from build123d import *

# Parameters (mm, degrees)
F1_DEPTH     = 25
F2_T         = 2
F3_T1_DEPTH  = 31
F3_T3_DEPTH  = 46
F3_T9_DEPTH  = 51
F3_T13_DEPTH = 36
F3_T20_DEPTH = 36
F3_T24_DEPTH = 51
F3_T31_DEPTH = 36
F3_T35_DEPTH = 51
F3_T42_DEPTH = 36
F3_T46_DEPTH = 51
F4_R         = 3
F5_R         = 1
F6_DEPTH     = 4
F8_W         = 10
F8_H         = 4
F9_DEPTH     = 4


# Not quite as in the source:
# - a fillet or chamfer that OpenCascade refuses, or shapes differently, is made with other operations: its cross-section is extruded or revolved along the edge and cut away or added
# - a shell that OpenCascade refuses in one call is made with other operations: the cavity is built on its own and cut out


with BuildPart() as f1:
    # F0 (on Top) → F1 (new body)
    with BuildSketch(Plane.XY):
        with BuildLine():
            ThreePointArc((25, 15.5), (24.4142135624, 16.9142135624), (23, 17.5))
            Line((23, 17.5), (-23, 17.5))
            ThreePointArc((-23, 17.5), (-24.4142135624, 16.9142135624), (-25, 15.5))
            Line((-25, 15.5), (-25, -15.5))
            ThreePointArc((-25, -15.5), (-24.4142135624, -16.9142135624), (-23, -17.5))
            Line((-23, -17.5), (23, -17.5))
            ThreePointArc((23, -17.5), (24.4142135624, -16.9142135624), (25, -15.5))
            Line((25, -15.5), (25, 15.5))
        make_face()
    extrude(amount=F1_DEPTH)

    # F2: shell of thickness 2, made by hand


with BuildPart() as f2_core1:
    # F2_t2: copy of F1
    add(f1.part)

    # the walls: a layer under each face that stays
    f2_faces = [f2_core1.faces().sort_by_distance(p)[0] for p in [
        (0, 17.5, 12.5),
        (-25, 0, 12.5),
        (0, -17.5, 12.5),
        (25, 0, 12.5),
        (0, 0, 0),
    ]]
    thicken(f2_faces, amount=-F2_T, mode=Mode.SUBTRACT)


with BuildPart() as f1_1:
    add(f1.part)

    # what is left inside the walls is the cavity
    f2_cavity = [f2_core1.part.solids().sort_by_distance(p)[0] for p in [
        (0, -5.166667, 2.02),
    ]]
    add(f2_cavity, mode=Mode.SUBTRACT)

    # F3: fillet of radius 2 on 4 edges, made by hand

    # F3_s2 → F3_t1 (cut)
    with BuildSketch(Plane.XZ.offset(-15.5)):
        with BuildLine():
            ThreePointArc((-25, 25), (-23.5857864376, 24.4142135624), (-23, 23))
            Line((-23, 23), (-22.96, 23))
            Line((-22.96, 23), (-22.96, 25.04))
            Line((-22.96, 25.04), (-25, 25.04))
            Line((-25, 25.04), (-25, 25))
        make_face()
        with BuildLine():
            ThreePointArc((25, 25), (23.5857864376, 24.4142135624), (23, 23))
            Line((23, 23), (22.96, 23))
            Line((22.96, 23), (22.96, 25.04))
            Line((22.96, 25.04), (25, 25.04))
            Line((25, 25.04), (25, 25))
        make_face()
    extrude(amount=F3_T1_DEPTH, mode=Mode.SUBTRACT)

    # F3_s4 → F3_t3 (cut)
    with BuildSketch(Plane.YZ.offset(-23)):
        with BuildLine():
            ThreePointArc((17.5, 25), (16.0857864376, 24.4142135624), (15.5, 23))
            Line((15.5, 23), (15.46, 23))
            Line((15.46, 23), (15.46, 25.04))
            Line((15.46, 25.04), (17.5, 25.04))
            Line((17.5, 25.04), (17.5, 25))
        make_face()
        with BuildLine():
            ThreePointArc((-17.5, 25), (-16.0857864376, 24.4142135624), (-15.5, 23))
            Line((-15.5, 23), (-15.46, 23))
            Line((-15.46, 23), (-15.46, 25.04))
            Line((-15.46, 25.04), (-17.5, 25.04))
            Line((-17.5, 25.04), (-17.5, 25))
        make_face()
    extrude(amount=F3_T3_DEPTH, mode=Mode.SUBTRACT)


with BuildPart() as f3_tool7:
    # F3_s8 → F3_t9 (new body)
    with BuildSketch(Plane.YZ.offset(23)):
        with BuildLine():
            ThreePointArc((17.5, 25), (16.0857864376, 24.4142135624), (15.5, 23))
            Line((15.5, 23), (15.46, 23))
            Line((15.46, 23), (15.46, 25.04))
            Line((15.46, 25.04), (17.5, 25.04))
            Line((17.5, 25.04), (17.5, 25))
        make_face()
    extrude(amount=-F3_T9_DEPTH)

    split(bisect_by=Plane.YZ.offset(-23), keep=Keep.BOTTOM)


with BuildPart() as f3_tool11:
    # F3_s12 → F3_t13 (new body)
    with BuildSketch(Plane.XZ.offset(-20.5)):
        with BuildLine():
            ThreePointArc((-25, 25), (-23.5857864376, 24.4142135624), (-23, 23))
            Line((-23, 23), (-22.96, 23))
            Line((-22.96, 23), (-22.96, 25.04))
            Line((-22.96, 25.04), (-25, 25.04))
            Line((-25, 25.04), (-25, 25))
        make_face()
    extrude(amount=F3_T13_DEPTH)

    split(bisect_by=Plane.XZ.offset(-15.5), keep=Keep.BOTTOM)


with BuildPart() as f3_tool7_1:
    add(f3_tool7.part)

    # F3_t15: intersect F3_tool11
    add(f3_tool11.part, mode=Mode.INTERSECT)


with BuildPart() as f1_2:
    add(f1_1.part)

    # F3_t5: cut F3_tool7
    add(f3_tool7_1.part, mode=Mode.SUBTRACT)


with BuildPart() as f3_tool18:
    # F3_s19 → F3_t20 (new body)
    with BuildSketch(Plane.XZ.offset(-15.5)):
        with BuildLine():
            ThreePointArc((-25, 25), (-23.5857864376, 24.4142135624), (-23, 23))
            Line((-23, 23), (-22.96, 23))
            Line((-22.96, 23), (-22.96, 25.04))
            Line((-22.96, 25.04), (-25, 25.04))
            Line((-25, 25.04), (-25, 25))
        make_face()
    extrude(amount=F3_T20_DEPTH)

    split(bisect_by=Plane.XZ.offset(15.5), keep=Keep.TOP)


with BuildPart() as f3_tool22:
    # F3_s23 → F3_t24 (new body)
    with BuildSketch(Plane.YZ.offset(-28)):
        with BuildLine():
            ThreePointArc((-17.5, 25), (-16.0857864376, 24.4142135624), (-15.5, 23))
            Line((-15.5, 23), (-15.46, 23))
            Line((-15.46, 23), (-15.46, 25.04))
            Line((-15.46, 25.04), (-17.5, 25.04))
            Line((-17.5, 25.04), (-17.5, 25))
        make_face()
    extrude(amount=F3_T24_DEPTH)

    split(bisect_by=Plane.YZ.offset(-23), keep=Keep.BOTTOM)


with BuildPart() as f3_tool18_1:
    add(f3_tool18.part)

    # F3_t26: intersect F3_tool22
    add(f3_tool22.part, mode=Mode.INTERSECT)


with BuildPart() as f1_3:
    add(f1_2.part)

    # F3_t16: cut F3_tool18
    add(f3_tool18_1.part, mode=Mode.SUBTRACT)


with BuildPart() as f3_tool29:
    # F3_s30 → F3_t31 (new body)
    with BuildSketch(Plane.XZ.offset(15.5)):
        with BuildLine():
            ThreePointArc((25, 25), (23.5857864376, 24.4142135624), (23, 23))
            Line((23, 23), (22.96, 23))
            Line((22.96, 23), (22.96, 25.04))
            Line((22.96, 25.04), (25, 25.04))
            Line((25, 25.04), (25, 25))
        make_face()
    extrude(amount=-F3_T31_DEPTH)

    split(bisect_by=Plane.XZ.offset(-15.5), keep=Keep.BOTTOM)


with BuildPart() as f3_tool33:
    # F3_s34 → F3_t35 (new body)
    with BuildSketch(Plane.YZ.offset(28)):
        with BuildLine():
            ThreePointArc((17.5, 25), (16.0857864376, 24.4142135624), (15.5, 23))
            Line((15.5, 23), (15.46, 23))
            Line((15.46, 23), (15.46, 25.04))
            Line((15.46, 25.04), (17.5, 25.04))
            Line((17.5, 25.04), (17.5, 25))
        make_face()
    extrude(amount=-F3_T35_DEPTH)

    split(bisect_by=Plane.YZ.offset(23), keep=Keep.TOP)


with BuildPart() as f3_tool29_1:
    add(f3_tool29.part)

    # F3_t37: intersect F3_tool33
    add(f3_tool33.part, mode=Mode.INTERSECT)


with BuildPart() as f1_4:
    add(f1_3.part)

    # F3_t27: cut F3_tool29
    add(f3_tool29_1.part, mode=Mode.SUBTRACT)


with BuildPart() as f3_tool40:
    # F3_s41 → F3_t42 (new body)
    with BuildSketch(Plane.XZ.offset(20.5)):
        with BuildLine():
            ThreePointArc((25, 25), (23.5857864376, 24.4142135624), (23, 23))
            Line((23, 23), (22.96, 23))
            Line((22.96, 23), (22.96, 25.04))
            Line((22.96, 25.04), (25, 25.04))
            Line((25, 25.04), (25, 25))
        make_face()
    extrude(amount=-F3_T42_DEPTH)

    split(bisect_by=Plane.XZ.offset(15.5), keep=Keep.TOP)


with BuildPart() as f3_tool44:
    # F3_s45 → F3_t46 (new body)
    with BuildSketch(Plane.YZ.offset(-23)):
        with BuildLine():
            ThreePointArc((-17.5, 25), (-16.0857864376, 24.4142135624), (-15.5, 23))
            Line((-15.5, 23), (-15.46, 23))
            Line((-15.46, 23), (-15.46, 25.04))
            Line((-15.46, 25.04), (-17.5, 25.04))
            Line((-17.5, 25.04), (-17.5, 25))
        make_face()
    extrude(amount=F3_T46_DEPTH)

    split(bisect_by=Plane.YZ.offset(23), keep=Keep.TOP)


with BuildPart() as f3_tool40_1:
    add(f3_tool40.part)

    # F3_t48: intersect F3_tool44
    add(f3_tool44.part, mode=Mode.INTERSECT)


with BuildPart() as f1_5:
    add(f1_4.part)

    # F3_t38: cut F3_tool40
    add(f3_tool40_1.part, mode=Mode.SUBTRACT)

    # F4
    f4_edges = [f1_5.edges().sort_by_distance(p)[0] for p in [
        (0, 15.5, 2),
        (23, 0, 2),
        (0, -15.5, 2),
        (-23, 0, 2),
    ]]
    fillet(f4_edges, radius=F4_R)

    # F5 (on Top) → F6 (join)
    with BuildSketch(Plane.XY):
        with Locations((-9, 4.5)):
            Circle(F5_R)
        with Locations((-9, -5.5)):
            Circle(F5_R)
        with Locations((9, 4.5)):
            Circle(F5_R)
        with Locations((9, -5.5)):
            Circle(F5_R)
    extrude(amount=F6_DEPTH)

    # F8 (on offset) → F9 (cut, symmetric)
    with BuildSketch(Plane.YZ.offset(23.5)):
        with Locations((0, 6)):
            Rectangle(F8_W, F8_H)
    extrude(amount=F9_DEPTH, both=True, mode=Mode.SUBTRACT)


solid = f1_5.part
Part model, mm, in its own coordinate system. A direction names the side the tool comes from. Round coordinates to 2 decimals unless told otherwise and drop trailing zeros. Loops run counter-clockwise (first coordinate to the right, second up) from the corner with the lowest first, then second, coordinate; pieces in that order, holes last. Notation, with made-up numbers: (29.5, 56) - (71.5, 56) arc R20 ccw to (71.5, 60) - close; hole circle Ø1 at (2, 52.5). An arc over 180 degrees is marked (long way). Answer as a JSON object with one key per item and string values.
Item 1: Pull direction X, two halves, no side cores. Call faces 4 (the face through (0.34, 16.1, 24.43)), 5 (the face through (-24.4, 16.93, 12.33)), 6 (the face through (25, 0, 12)): pulls with the +X half, pulls with the -X half, needs draft (parallel to the pull), parting line crosses it, or undercut.
Output:
{"face 4": "undercut", "face 5": "pulls with the -X half", "face 6": "pulls with the +X half"}
Item 2: Band-saw the part on D-D on y = 11. List the corners of the cut face in (x, z).
Output:
{"outline": "(-25, 0) - (25, 0) - (25, 25) arc R2 ccw to (23, 23) - (23, 5) arc R3 cw to (20, 2) - (-20, 2) arc R3 cw to (-23, 5) - (-23, 23) arc R2 ccw to (-25, 25) - close"}
Item 3: Band-saw the part on B-B on z = 13.5. List the corners of the cut face in (x, y).
Output:
{"outline": "(-25, -15.5) arc R2 ccw to (-23, -17.5) - (23, -17.5) arc R2 ccw to (25, -15.5) - (25, 15.5) arc R2 ccw to (23, 17.5) - (-23, 17.5) arc R2 ccw to (-25, 15.5) - close; hole (-23, -15.5) - (23, -15.5) - (23, 15.5) - (-23, 15.5) - close"}
Item 4: Pin check, flat tips, straight feed: pin 1 (12.5 mm diameter, centred on x = 3.5, y = -5, fed in from +Z); pin 2 (1.1 mm diameter, centred on x = 23.5, y = -0.5, fed in from +Z); pin 3 (0.7 mm diameter, centred on x = 24, z = 5.5, fed in from -Y). Stop position of each tip, or through.
Output:
{"pin 1": "z = 4", "pin 2": "z = 24.76", "pin 3": "y = -17.39"}
Item 5: Wall check: L1, parallel to X at y = -8, z = 10; L2, parallel to Y at x = -20.5, z = 16.25; L3, parallel to Z at x = -12, y = 2. Give the ranges that are in metal, low to high.
Output:
{"L1": "-25 to -23, 23 to 25", "L2": "-17.5 to -15.5, 15.5 to 17.5", "L3": "0 to 2"}
Item 6: Tool access for faces 1 (the face through (24, 5, 6)), 2 (the face through (-0.32, 14.64, 2.9)), 3 (the face through (0, -17.5, 12)): list every direction of +Z, -Z, +X, -X, +Y, -Y with a clear straight run to the whole face (end or side of a thin tool).
Output:
{"face 1": "+X", "face 2": "+Z", "face 3": "+Z, -Z, +X, -X, -Y"}
Item 7: Band-saw the part on A-A on y = -1. List the corners of the cut face in (x, z).
Output:
{"outline": "(-25, 0) - (25, 0) - (25, 4) - (22.83, 4) arc R3 cw to (20, 2) - (-20, 2) arc R3 cw to (-23, 5) - (-23, 23) arc R2 ccw to (-25, 25) - close; (23, 8) - (25, 8) - (25, 25) arc R2 ccw to (23, 23) - close"}
Item 8: Band-saw the part on C-C on x = -4. List the corners of the cut face in (y, z), plus the area to 3 significant figures.
Output:
{"outline": "(-17.5, 0) - (17.5, 0) - (17.5, 25) arc R2 ccw to (15.5, 23) - (15.5, 5) arc R3 cw to (12.5, 2) - (-12.5, 2) arc R3 cw to (-15.5, 5) - (-15.5, 23) arc R2 ccw to (-17.5, 25) - close", "area": "164 mm2"}
